from build123d import *

# Parameters (mm, degrees)
SKETCH1_R           = 4
BOSS_EXTRUDE1_DEPTH = 16.5
CUT_EXTRUDE1_START  = -8.68
CUT_EXTRUDE1_DEPTH  = 8.68
SKETCH5_R           = 2
CUT_EXTRUDE3_DEPTH  = 7
SKETCH4_R           = 1.275
SKETCH4_R_2         = 1.27
CUT_EXTRUDE2_DEPTH  = 18.846568298
FILLET1_R           = 1


with BuildPart() as part:
    # Sketch1 → Boss-Extrude1 (new body)
    with BuildSketch(Plane(origin=(0, 0, 0), x_dir=(1, 0, 0), z_dir=(0, 1, 0))):
        with Locations(Location((0, 0, 0), (0, 0, 270))):
            Circle(SKETCH1_R)
    extrude(amount=BOSS_EXTRUDE1_DEPTH)

    # Sketch2 → Cut-Extrude1 (cut)
    with BuildSketch(Plane(origin=(0, 16.5, 0), x_dir=(1, 0, 0), z_dir=(0, 1, 0)).offset(CUT_EXTRUDE1_START)):
        with BuildLine():
            Line((-3.708099244, 1.5), (3.708099244, 1.5))
            ThreePointArc((3.708099244, 1.5), (0, 4), (-3.708099244, 1.5))
        make_face()
        with BuildLine():
            Line((-3.708099244, -1.5), (3.708099244, -1.5))
            ThreePointArc((3.708099244, -1.5), (0, -4), (-3.708099244, -1.5))
        make_face()
    extrude(amount=CUT_EXTRUDE1_DEPTH, mode=Mode.SUBTRACT)

    # Sketch5 → Cut-Extrude3 (cut)
    with BuildSketch(Plane.XZ):
        with Locations(Location((0, 0, 0), (0, 0, 270))):
            Circle(SKETCH5_R)
    extrude(amount=-CUT_EXTRUDE3_DEPTH, mode=Mode.SUBTRACT)

    # Sketch4 → Cut-Extrude2 (cut, through all)
    with BuildSketch(Plane.XY.offset(1.5)):
        with Locations((0, 13.965)):
            Circle(SKETCH4_R)
        with Locations(Location((0, 4.72, 0), (0, 0, 90))):
            Circle(SKETCH4_R_2)
    extrude(amount=-CUT_EXTRUDE2_DEPTH, mode=Mode.SUBTRACT)

    # Fillet1
    fillet1_edges = [part.edges().sort_by_distance(p)[0] for p in [
        (4, 16.5, 0),
        (-4, 16.5, 0),
    ]]
    fillet(fillet1_edges, radius=FILLET1_R)


solid = part.part
Work out the finished part from the listing and answer in its coordinate system (mm). A direction names the side the tool comes from. Round coordinates to 2 decimals unless told otherwise and drop trailing zeros. Loops run counter-clockwise (first coordinate to the right, second up) from the corner with the lowest first, then second, coordinate; pieces in that order, holes last. Notation, with made-up numbers: M 13.25,-8 L 60.25,-8 A36 cw 60.25,26 Z; hole C 11.5,57.25 d2. An arc over 180 degrees is marked long. One line per question, with ' | ' between items. Start each with the question number.
(1) A tool of negligible diameter and unlimited length cuts with its end or side. For faces 5 (the face through (0, 12, -1.5)), 6 (the face through (0, 3, 2)), 7 (the face through (-0.06, 3.45, -2.76)), 8 (the face through (-1, 0, -2)), from which of +Z, -Z, +X, -X, +Y, -Y can it reach the whole face along a straight path? Write none if from no direction.
(2) A cutting plane is placed at D-D on x = 1.5. Write down the section's boundary in (y, z).
(3) Find the intervals of material crossed by line 1 (X direction, y = 5.25, z = 0); line 2 (Y direction, x = 0, z = -2.2); line 3 (Z direction, x = 3, y = 13.25), in increasing order.
(4) A cutting plane is placed at B-B on y = 3.25. Write down the section's boundary in (x, z), plus the area to 3 significant figures.
(5) For a pull along Z with two mould halves and no side action, classify faces 1 (the face through (0, 7, 0)), 2 (the face through (0, 7.82, 2)), 3 (the face through (0, 12, 1.5)), 4 (the face through (1.201, 5.919, 3.815)) as released by +Z, released by -Z, zero draft, split by the parting line, or undercut.
(6) Flat-ended cylindrical pins translate along their axes: pin 1 Ø4.5 at (x, z) = (0, 0) entering from -Y; pin 2 Ø2 at (x, z) = (-1.5, 3) entering from +Y; pin 3 Ø3.5 at (x, y) = (0.5, 10.5) entering from +Z; pin 4 Ø4 at (x, y) = (0, 13.965) entering from -Z. Find the tip coordinate at first contact, or state that the pin passes through.
(7) A cutting plane is placed at C-C on z = 0. Write down the section's boundary in (x, y) (3 decimals).
(8) A cutting plane is placed at A-A on x = 0. Write down the section's boundary in (y, z), plus the area to 3 significant figures.
Geometry check:
1) face 5: -Z, +X, -X, +Y | face 6: -Y | face 7: -Z | face 8: +Z, -Z, +X, -X, -Y
2) outline: M 0,-3.71 L 7.82,-3.71 L 7.82,-1.5 L 16.5,-1.5 L 16.5,1.5 L 7.82,1.5 L 7.82,3.71 L 0,3.71 L 0,1.32 L 7,1.32 L 7,-1.32 L 0,-1.32 Z
3) line 1: x = -4 to -2, 2 to 4 | line 2: y = 0 to 3.45, 5.99 to 7.82 | line 3: z = -1.5 to 1.5
4) outline: C 0,0 d8; hole C 0,0 d4 | area: 37.7 mm²
5) face 1: undercut | face 2: zero draft | face 3: released by +Z | face 4: split by the parting line
6) pin 1: stops at y = 0 | pin 2: stops at y = 7.82 | pin 3: stops at z = 1.5 | pin 4: stops at z = -1.5
7) outline: M -4,0 L -2,0 L -2,7 L 2,7 L 2,0 L 4,0 L 4,15.5 A1 ccw 3,16.5 L -3,16.5 A1 ccw -4,15.5 Z; hole C 0,13.965 d2.55
8) outline: M 0,-4 L 3.45,-4 L 3.45,-2 L 0,-2 Z; M 0,2 L 7,2 L 7,-2 L 5.99,-2 L 5.99,-4 L 7.82,-4 L 7.82,-1.5 L 12.69,-1.5 L 12.69,1.5 L 7.82,1.5 L 7.82,4 L 0,4 Z; M 15.24,-1.5 L 16.5,-1.5 L 16.5,1.5 L 15.24,1.5 Z | area: 47.9 mm²
